Part model, mm, in its own coordinate system. A direction names the side the tool comes from. Round coordinates to 2 decimals unless told otherwise and drop trailing zeros. Order: outer loops, then holes, each group sorted by start corner. A loop starts at its lowest first (then second) coordinate and runs counter-clockwise, first axis right, second up. Notation, with made-up numbers: (8.5, 64.5) - (63.5, 64.5) arc R26 cw to (63.5, 97.5) - close; hole circle Ø11 at (49.5, 60). An arc over 180 degrees is marked (long way). Answer as a JSON object with one key per item and string values.
```python
from build123d import *

# Parameters (mm, degrees)
F0_R     = 14.2875
F1_DEPTH = 25.4
F2_DEPTH = 50.8
F3_DEPTH = 50.8


with BuildPart() as f1:
    # F0 (on Front) → F1 (new body)
    with BuildSketch(Plane.XZ):
        with BuildLine():
            ThreePointArc((5.211817, -28.095686), (21.971098, -18.270235), (28.575, 0))
            ThreePointArc((28.575, 0), (21.971098, 18.270235), (5.211817, 28.095686))
            ThreePointArc((5.211817, 28.095686), (-28.575, 0), (5.211817, -28.095686))
        make_face()
        with BuildLine():
            ThreePointArc((-13.470384, 4.7625), (0, 14.2875), (13.470384, 4.7625))
            Line((13.470384, 4.7625), (19.05, 4.7625))
            Line((19.05, 4.7625), (19.05, -4.7625))
            Line((19.05, -4.7625), (13.470384, -4.7625))
            ThreePointArc((13.470384, -4.7625), (0, -14.2875), (-13.470384, -4.7625))
            Line((-13.470384, -4.7625), (-19.05, -4.7625))
            Line((-19.05, -4.7625), (-19.05, 4.7625))
            Line((-19.05, 4.7625), (-13.470384, 4.7625))
        make_face(mode=Mode.SUBTRACT)
        with BuildLine():
            ThreePointArc((5.211817, 28.095686), (21.971098, 18.270235), (28.575, 0))
            ThreePointArc((28.575, 0), (21.971098, -18.270235), (5.211817, -28.095686))
            Line((5.211817, -28.095686), (53.975, -19.05))
            ThreePointArc((53.975, -19.05), (34.925, 0), (53.975, 19.05))
            Line((53.975, 19.05), (5.211817, 28.095686))
        make_face()
        with BuildLine():
            ThreePointArc((73.025, 0), (67.445384, 13.470384), (53.975, 19.05))
            ThreePointArc((53.975, 19.05), (34.925, 0), (53.975, -19.05))
            ThreePointArc((53.975, -19.05), (67.445384, -13.470384), (73.025, 0))
        make_face()
        with Locations((53.975, 0)):
            Circle(F0_R, mode=Mode.SUBTRACT)
    extrude(amount=F1_DEPTH)

    # F0 (on Front) → F2 (join)
    with BuildSketch(Plane.XZ):
        with BuildLine():
            ThreePointArc((5.211817, -28.095686), (21.971098, -18.270235), (28.575, 0))
            ThreePointArc((28.575, 0), (21.971098, 18.270235), (5.211817, 28.095686))
            ThreePointArc((5.211817, 28.095686), (-28.575, 0), (5.211817, -28.095686))
        make_face()
        with BuildLine():
            ThreePointArc((-13.470384, 4.7625), (0, 14.2875), (13.470384, 4.7625))
            Line((13.470384, 4.7625), (19.05, 4.7625))
            Line((19.05, 4.7625), (19.05, -4.7625))
            Line((19.05, -4.7625), (13.470384, -4.7625))
            ThreePointArc((13.470384, -4.7625), (0, -14.2875), (-13.470384, -4.7625))
            Line((-13.470384, -4.7625), (-19.05, -4.7625))
            Line((-19.05, -4.7625), (-19.05, 4.7625))
            Line((-19.05, 4.7625), (-13.470384, 4.7625))
        make_face(mode=Mode.SUBTRACT)
    extrude(amount=F2_DEPTH)

    # F0 (on Front) → F3 (join)
    with BuildSketch(Plane.XZ):
        with BuildLine():
            ThreePointArc((-13.470384, -4.7625), (-14.2875, 0), (-13.470384, 4.7625))
            Line((-13.470384, 4.7625), (-19.05, 4.7625))
            Line((-19.05, 4.7625), (-19.05, -4.7625))
            Line((-19.05, -4.7625), (-13.470384, -4.7625))
        make_face()
    extrude(amount=F3_DEPTH)


solid = f1.part
```
Item 1: Cut at C-C (z = -6.5). Write the cut outline in (x, y), plus the area to 3 significant figures.
Taken from the geometry:
{"outline": "(-27.83, -50.8) - (-12.72, -50.8) - (-12.72, 0) - (-27.83, 0) - close; (12.72, -50.8) - (27.83, -50.8) - (27.83, -25.4) - (41.25, -25.4) - (41.25, 0) - (12.72, 0) - close; (66.7, -25.4) - (71.88, -25.4) - (71.88, 0) - (66.7, 0) - close", "area": "2,010 mm2"}
Item 2: Probe L1, parallel to Z at x = 54.5, y = -24; L2, parallel to Y at x = 34, z = -21.5; L3, parallel to Z at x = 16, y = -16.5. List the from-to ranges inside material, lowest first. Write a range as from..to.
Taken from the geometry:
{"L1": "-19.04..-14.28, 14.28..19.04", "L2": "-25.4..0", "L3": "-26.09..-4.76, 4.76..26.09"}
Item 3: Tool access for faces 4 (the flat face through (22, 0, 0)), 5 (the flat face through (16, -25, 4.762)): list every direction of +Z, -Z, +X, -X, +Y, -Y with a clear straight run to the whole face (end or side of a thin tool).
Taken from the geometry:
{"face 4": "+Z, -Z, +X, -X, +Y", "face 5": "+Y, -Y"}
Item 4: Two-plate mould, pull along X, no slides. Class faces 1 (the flat face through (16, -25, -4.762)), 2 (the flat face through (39, -25.4, 2)), 3 (the flat face through (29.252, -12.522, -23.636)): pulls with the +X half, pulls with the -X half, needs draft (parallel to the pull), parting line crosses it, or undercut.
Taken from the geometry:
{"face 1": "undercut", "face 2": "needs draft", "face 3": "pulls with the +X half"}
Item 5: Cut at A-A (x = 0). Write the cut outline in (y, z) (1 decimal).
Taken from the geometry:
{"outline": "(-50.8, -28.6) - (0, -28.6) - (0, -14.3) - (-50.8, -14.3) - close; (-50.8, 14.3) - (0, 14.3) - (0, 28.6) - (-50.8, 28.6) - close"}
Item 6: Cut at B-B (y = -11). State how many separate pieces and enclosed holes the cut face has, plus the area to 3 significant figures.
Taken from the geometry:
{"separate pieces": "1", "enclosed holes": "2", "area": "3,120 mm2"}
Item 7: Drop flat-ended pins along their axis: P1, Ø3, axis at y = -30, z = -1, coming from the +X side (3 decimals); P2, Ø1.5, axis at x = 22, y = -15, coming from the -Z side; P3, Ø8, axis at x = 59, y = -19, coming from the -Z side. Give the stop position or say it passes through.
Taken from the geometry:
{"P1": "x = 28.575", "P2": "z = -25.12", "P3": "z = -19.02"}
